```python
from build123d import *

# Parameters (mm, degrees)
SKETCH1_R           = 1.8288
BOSS_EXTRUDE1_DEPTH = 6.35


with BuildPart() as part:
    # Sketch1 → Boss-Extrude1 (new body)
    with BuildSketch(Plane(origin=(0, 0, 0), x_dir=(1, 0, 0), z_dir=(0, 1, 0))):
        Polygon((-48.0314, 76.2), (48.0314, 76.2), (48.0314, 60.325), (-28.1686, 60.325), (-28.1686, 53.975), (48.0314, 53.975), (48.0314, 22.225), (-28.1686, 22.225), (-28.1686, 15.875), (48.0314, 15.875), (48.0314, -15.875), (-28.1686, -15.875), (-28.1686, -22.225), (48.0314, -22.225), (48.0314, -53.975), (-28.1686, -53.975), (-28.1686, -60.325), (48.0314, -60.325), (48.0314, -76.2), (-48.0314, -76.2), (-48.0314, -39.9288), (-44.3484, -39.9288), (-44.3484, -42.037), (-41.6814, -42.037), (-41.6814, -34.163), (-44.3484, -34.163), (-44.3484, -36.2712), (-48.0314, -36.2712), (-48.0314, -1.8288), (-44.3484, -1.8288), (-44.3484, -3.937), (-41.6814, -3.937), (-41.6814, 3.937), (-44.3484, 3.937), (-44.3484, 1.8288), (-48.0314, 1.8288), (-48.0314, 36.2712), (-44.3484, 36.2712), (-44.3484, 34.163), (-41.6814, 34.163), (-41.6814, 42.037), (-44.3484, 42.037), (-44.3484, 39.9288), (-48.0314, 39.9288), align=None)
        with Locations((-38.1, 57.15)):
            Circle(SKETCH1_R, mode=Mode.SUBTRACT)
        with Locations((-38.1, 19.05)):
            Circle(SKETCH1_R, mode=Mode.SUBTRACT)
        with Locations((-38.1, -19.05)):
            Circle(SKETCH1_R, mode=Mode.SUBTRACT)
        with Locations((-38.1, -57.15)):
            Circle(SKETCH1_R, mode=Mode.SUBTRACT)
    extrude(amount=-BOSS_EXTRUDE1_DEPTH)


solid = part.part
```
Read the model definition and answer for the solid it produces. Units are mm, in the model's axes. A direction names the side the tool comes from. Give positions to 0.01 mm unless a question says otherwise; leave off trailing zeros. Order: outer loops, then holes, each group sorted by start corner. A loop starts at its lowest first (then second) coordinate and runs counter-clockwise, first axis right, second up.
(1) Find section A-A (x = -8.5). Give the vertices of the cut face in (y, z) (3 decimals), plus the area to 3 significant figures.
(2) For faces 1 (the flat face through (48.031, -3, -38)), 2 (the flat face through (-46, -3, 1.829)), 3 (the flat face through (-41.681, -3, 0)), 4 (the flat face through (-28.169, -3, -57)), determine the directions among +Z, -Z, +X, -X, +Y, -Y from which every point of the face is accessible in a straight line to the end or side of a thin tool.
(3) For a pull along X with two mould halves and no side action, classify faces 5 (the flat face through (-48.031, -3, -19)), 6 (the flat face through (-46, -3, -39.929)), 7 (the flat face through (-41.681, -3, -38)), 8 (the flat face through (48.031, -3, 0)) as released by +X, released by -X, zero draft, split by the parting line, or undercut.
(4) Given pin 1 (1.9 mm diameter, centred on y = -1.5, z = -55.5, fed in from +X), flat-ended and moving along its own axis, determine where the tip first touches the part or whether it passes through.
(5) Straight lines are drawn through the part: L1, parallel to Z at x = -43, y = -1.75; L2, parallel to Z at x = -38, y = -6; L3, parallel to Z at x = -18, y = -2.25 (3 decimals). For each, find the intervals that lie inside material, in ascending order.
(6) Find section B-B (z = 19.05). Give the vertices of the cut face in (x, y), plus the area to 3 significant figures.
(7) Find section C-C (x = -38.1). Give the vertices of the cut face in (y, z), plus the area to 3 significant figures.
(8) Find section D-D (y = -4.75). Give the number of separate pieces and of enclosed holes in the cut face, plus the area to 3 significant figures.
Result sheet:
1. outline: (-6.35, -76.2) - (0, -76.2) - (0, -60.325) - (-6.35, -60.325) - close; (-6.35, -53.975) - (0, -53.975) - (0, -22.225) - (-6.35, -22.225) - close; (-6.35, -15.875) - (0, -15.875) - (0, 15.875) - (-6.35, 15.875) - close; (-6.35, 22.225) - (0, 22.225) - (0, 53.975) - (-6.35, 53.975) - close; (-6.35, 60.325) - (0, 60.325) - (0, 76.2) - (-6.35, 76.2) - close
1. area: 806 mm2
2. face 1: +Z, -Z, +X, +Y, -Y
2. face 2: -X, +Y, -Y
2. face 3: +Y, -Y
2. face 4: +X, +Y, -Y
3. face 5: released by -X
3. face 6: zero draft
3. face 7: undercut
3. face 8: released by +X
4. pin 1: stops at x = -28.17
5. L1: z = -76.2 to -42.04, -34.16 to -3.94, 3.94 to 34.16, 42.04 to 76.2
5. L2: z = -76.2 to -58.98, -55.32 to -20.88, -17.22 to 17.22, 20.88 to 55.32, 58.98 to 76.2
5. L3: z = -76.2 to -60.325, -53.975 to -22.225, -15.875 to 15.875, 22.225 to 53.975, 60.325 to 76.2
6. outline: (-48.03, -6.35) - (-39.93, -6.35) - (-39.93, 0) - (-48.03, 0) - close; (-36.27, -6.35) - (-28.17, -6.35) - (-28.17, 0) - (-36.27, 0) - close
6. area: 103 mm2
7. outline: (-6.35, -76.2) - (0, -76.2) - (0, -58.98) - (-6.35, -58.98) - close; (-6.35, -55.32) - (0, -55.32) - (0, -20.88) - (-6.35, -20.88) - close; (-6.35, -17.22) - (0, -17.22) - (0, 17.22) - (-6.35, 17.22) - close; (-6.35, 20.88) - (0, 20.88) - (0, 55.32) - (-6.35, 55.32) - close; (-6.35, 58.98) - (0, 58.98) - (0, 76.2) - (-6.35, 76.2) - close
7. area: 875 mm2
8. separate pieces: 1
8. enclosed holes: 4
8. area: 12,600 mm2
